Can you work these out from the model? Positions are in its coordinate system, mm. Face numbers are marked on the shaded views. A direction names the side the tool comes from. Coordinates: 2 decimals unless noted, no trailing zeros. Order: outer loops, then holes, each group sorted by start corner. A loop starts at its lowest first (then second) coordinate and runs counter-clockwise, first axis right, second up. Notation, with made-up numbers: (73, -0.5) -> (82, -0.5) arc R18 cw to (82, 8.5) -> close; hole circle Ø9 at (-1.5, 87.5). An arc over 180 degrees is marked (long way). Use a Markdown table: item, result. Add a question column.
1. We'd pull the mould along Z, two halves only. Please class the marked faces 6, 7 and 8: pulls with the +Z half, pulls with the -Z half, needs draft (parallel to the pull), parting line crosses it, or undercut.
2. For the marked faces 1, 2, 3, 4 and 5, which set-ups out of +Z, -Z, +X, -X, +Y, -Y let a thin tool reach every point of the face, with its end or its side?
3. For pin 1 Ø17 at (x, y) = (32, 63) entering from +Z; pin 2 Ø5 at (x, y) = (13, 65) entering from +Z; pin 3 Ø22 at (y, z) = (37, -81) entering from +X, each with a flat end and sliding along its axis, tell me the tip position at first contact or that it passes through.
4. Suppose I cut it at A-A, the plane z = -102. List the corners of the cut face in (x, y) for me, then the cut area to 3 significant figures.
5. If I drill on line 1 along Y through (x, z) = (32, -73.75); line 2 along X through (y, z) = (83, 29.5); line 3 along Z through (x, y) = (44, 54.5), over which ranges is the centre line in solid material (lowest first)? Write a range as from..to.
6. Suppose I cut it at D-D, the plane x = 8.5. List the corners of the cut face in (y, z) for me, then the cut area to 3 significant figures.
7. Suppose I cut it at B-B, the plane x = 46. List the corners of the cut face in (y, z) for me, then the cut area to 3 significant figures.
8. Suppose I cut it at C-C, the plane y = 11.5. List the corners of the cut face in (x, z) for me.
```python
from build123d import *

# Parameters (mm, degrees)
EXTRUDE_THIN1_DEPTH     = 64
BOSS_EXTRUDE1_DEPTH     = 18
SKETCH3_W               = 61
SKETCH3_H               = 44
BOSS_EXTRUDE2_DEPTH     = 19
SKETCH4_W               = 29
SKETCH4_H               = 25
CUT_EXTRUDE1_DEPTH      = 191.964551072
CUT_EXTRUDE2_DEPTH      = 55
CUT_EXTRUDE2_DEPTH_BACK = 204.633149969
SKETCH5_R               = 19
SKETCH6_R               = 19
BOSS_EXTRUDE3_DEPTH     = 19
SKETCH8_R               = 19
BOSS_EXTRUDE4_DEPTH     = 19
SKETCH9_R               = 9.5
CUT_EXTRUDE3_DEPTH      = 171.817035937
CUT_EXTRUDE8_DEPTH      = 211.703583263
SKETCH16_W              = 22
SKETCH16_H              = 80
CUT_EXTRUDE9_DEPTH      = 6
SKETCH17_R              = 16
CUT_EXTRUDE10_DEPTH     = 6
SKETCH18_R              = 9.5
CUT_EXTRUDE11_DEPTH     = 19
SKETCH19_R              = 6.5
CUT_EXTRUDE12_DEPTH     = 19


with BuildPart() as part:
    # Sketch1 → Extrude-Thin1 (new body)
    with BuildSketch(Plane(origin=(0, 0, 0), x_dir=(0, 0, -1), z_dir=(1, 0, 0))):
        Polygon((-45, 77.942286341), (0, 0), (140, 0), (140, 19), (10.969655115, 19), (-28.545517328, 87.442286341), align=None)
    extrude(amount=EXTRUDE_THIN1_DEPTH)

    # Sketch2 → Boss-Extrude1 (add)
    with BuildSketch(Plane(origin=(0, 77.942286341, 45), x_dir=(1, 0, 0), z_dir=(0, 0.8660254037844362, 0.5000000000000046))):
        with BuildLine():
            Line((0, 0), (0, 51))
            ThreePointArc((0, 51), (32, 83), (64, 51))
            Line((64, 51), (64, 0))
            Line((64, 0), (0, 0))
        make_face()
    extrude(amount=-BOSS_EXTRUDE1_DEPTH)

    # Sketch3 → Boss-Extrude2 (add, symmetric)
    with BuildSketch(Plane(origin=(32, 0, 0), x_dir=(0, 0, -1), z_dir=(1, 0, 0))):
        with Locations((92.5, 41)):
            Rectangle(SKETCH3_W, SKETCH3_H)
    extrude(amount=BOSS_EXTRUDE2_DEPTH, both=True)

    # Sketch4 → Cut-Extrude1 (cut, through all)
    with BuildSketch(Plane(origin=(51, 0, 0), x_dir=(0, 0, -1), z_dir=(1, 0, 0))):
        with Locations((92.5, 50.5)):
            Rectangle(SKETCH4_W, SKETCH4_H)
    extrude(amount=-CUT_EXTRUDE1_DEPTH, mode=Mode.SUBTRACT)

    # Sketch5 → Cut-Extrude2 (cut, two sides: drawn at the far end of the back side and taken through both)
    with BuildSketch(Plane.XY.offset(-107).offset(-CUT_EXTRUDE2_DEPTH_BACK)):
        with Locations((32, 63)):
            Circle(SKETCH5_R)
    extrude(amount=CUT_EXTRUDE2_DEPTH + CUT_EXTRUDE2_DEPTH_BACK, mode=Mode.SUBTRACT)

    # Sketch6 → Boss-Extrude3 (add)
    with BuildSketch(Plane.XY.offset(-107)):
        with Locations((32, 63)):
            Circle(SKETCH6_R)
    extrude(amount=-BOSS_EXTRUDE3_DEPTH)

    # Sketch8 → Boss-Extrude4 (add)
    with BuildSketch(Plane(origin=(0, 0, -78), x_dir=(-1, 0, 0), z_dir=(0, 0, -1))):
        with Locations(Location((-32, 63, 0), (0, 0, 180))):
            Circle(SKETCH8_R)
    extrude(amount=-BOSS_EXTRUDE4_DEPTH)

    # Sketch9 → Cut-Extrude3 (cut, through all)
    with BuildSketch(Plane.XY.offset(-59)):
        with Locations((32, 63)):
            Circle(SKETCH9_R)
    extrude(amount=-CUT_EXTRUDE3_DEPTH, mode=Mode.SUBTRACT)

    # Sketch15 → Cut-Extrude8 (cut, through all)
    with BuildSketch(Plane(origin=(0, 77.942286341, 45), x_dir=(1, 0, 0), z_dir=(0, 0.8660254037844362, 0.5000000000000046))):
        Polygon((11, 0), (14.464101615, 6), (49.535898385, 6), (53, 0), align=None)
    extrude(amount=-CUT_EXTRUDE8_DEPTH, mode=Mode.SUBTRACT)

    # Sketch16 → Cut-Extrude9 (cut)
    with BuildSketch(Plane(origin=(0, 77.942286341, 45), x_dir=(1, 0, 0), z_dir=(0, 0.8660254037844362, 0.5000000000000046))):
        with Locations((32.014101615, 46)):
            Rectangle(SKETCH16_W, SKETCH16_H)
    extrude(amount=-CUT_EXTRUDE9_DEPTH, mode=Mode.SUBTRACT)

    # Sketch17 → Cut-Extrude10 (cut)
    with BuildSketch(Plane(origin=(0, 77.942286341, 45), x_dir=(1, 0, 0), z_dir=(0, 0.8660254037844362, 0.5000000000000046))):
        with Locations((32.014101615, 57)):
            Circle(SKETCH17_R)
    extrude(amount=-CUT_EXTRUDE10_DEPTH, mode=Mode.SUBTRACT)

    # Sketch18 → Cut-Extrude11 (cut)
    with BuildSketch(Plane(origin=(0, 72.746133918, 42), x_dir=(1, 0, 0), z_dir=(0, 0.866025403784436, 0.5000000000000047))):
        with Locations(Location((32.014101615, 57, 0), (0, 0, 270))):
            Circle(SKETCH18_R)
    extrude(amount=-CUT_EXTRUDE11_DEPTH, mode=Mode.SUBTRACT)

    # Sketch19 → Cut-Extrude12 (cut)
    with BuildSketch(Plane(origin=(0, 3, -5.196152423), x_dir=(1, 0, 0), z_dir=(0, -0.5000000000000044, 0.8660254037844362))):
        with Locations(Location((32.014101615, 56, 0), (0, 0, 270))):
            Circle(SKETCH19_R)
        with Locations(Location((32.014101615, 27, 0), (0, 0, 270))):
            Circle(SKETCH19_R)
    extrude(amount=-CUT_EXTRUDE12_DEPTH, mode=Mode.SUBTRACT)


solid = part.part
```
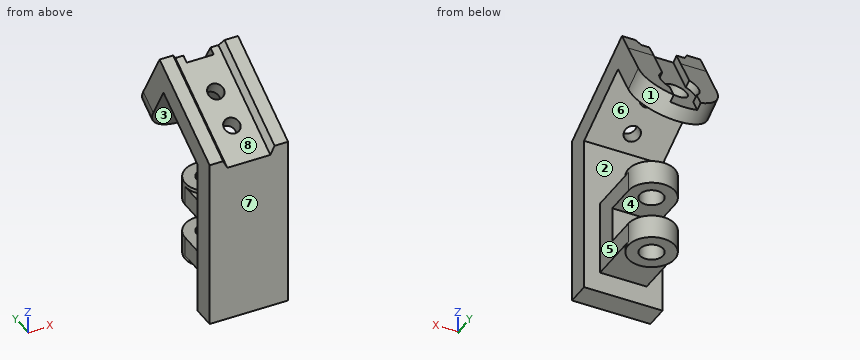
Worked out:
| question | item | result |
|---|---|---|
| 1 | face 6 | undercut |
| 1 | face 7 | needs draft |
| 1 | face 8 | pulls with the +Z half |
| 2 | face 1 | -Z, +Y |
| 2 | face 2 | none |
| 2 | face 3 | +X, -X |
| 2 | face 4 | +X, -X, +Y |
| 2 | face 5 | -Z, +X, +Y |
| 3 | pin 1 | stops at z = 34.35 |
| 3 | pin 2 | stops at z = 38.39 |
| 3 | pin 3 | stops at x = 51 |
| 4 | outline | (0, 0) -> (64, 0) -> (64, 19) -> (51, 19) -> (51, 38) -> (13, 38) -> (13, 19) -> (0, 19) -> close |
| 4 | area | 1,940 mm² |
| 5 | line 1 | y = 0..53.5, 72.5..82 |
| 5 | line 2 | x = 0..21.01, 43.01..64 |
| 5 | line 3 | z = -126..-107, -78..-59, 9.53..24.54 |
| 6 | outline | (0, -140) -> (19, -140) -> (19, -10.97) -> (71.85, 19.55) -> (98.71, -26.98) -> (114.3, -17.98) -> (77.94, 45) -> (0, 0) -> close |
| 6 | area | 5,130 mm² |
| 7 | outline | (0, -140) -> (19, -140) -> (19, -123) -> (50.15, -123) -> (50.15, -126) -> (75.85, -126) -> (75.85, -107) -> (38, -107) -> (38, -78) -> (75.85, -78) -> (75.85, -59) -> (50.15, -59) -> (50.15, -62) -> (19, -62) -> (19, -10.97) -> (71.85, 19.55) -> (102.24, -33.09) -> (117.83, -24.09) -> (110.33, -11.09) -> (105.13, -14.09) -> (97.36, -0.63) -> (102.56, 2.37) -> (80.94, 39.8) -> (0, -6.93) -> close |
| 7 | area | 7,140 mm² |
| 8 | outline | (0, -140) -> (64, -140) -> (64, 6.64) -> (53, 6.64) -> (49.54, -0.29) -> (14.46, -0.29) -> (11, 6.64) -> (0, 6.64) -> close |
